from build123d import *

# Parameters (mm, degrees)
SKETCH_1_W          = 40
SKETCH_1_H          = 63
EXTRUDE_1_DEPTH     = 16
SKETCH_2_W          = 38
SKETCH_2_H          = 61
CUT_EXTRUDE_2_DEPTH = 15
FILLET_2_R          = 1
SKETCH_5_W          = 38
SKETCH_5_H          = 2
CUT_EXTRUDE_4_DEPTH = 0.5
SKETCH_6_W          = 61.5
SKETCH_6_H          = 2
CUT_EXTRUDE_5_DEPTH = 0.5
SKETCH_7_W          = 38.5
SKETCH_7_H          = 2
CUT_EXTRUDE_6_DEPTH = 0.5
SKETCH_8_W          = 62
SKETCH_8_H          = 2
CUT_EXTRUDE_7_DEPTH = 0.5


with BuildPart() as part:
    # Эскиз1 → Бобышка-Вытянуть1 (new body)
    with BuildSketch(Plane(origin=(0, 0, 0), x_dir=(1, 0, 0), z_dir=(0, 1, 0))):
        with Locations((18.915, -30.961)):
            Rectangle(SKETCH_1_W, SKETCH_1_H)
    extrude(amount=EXTRUDE_1_DEPTH)

    # Эскиз2 → Вырез-Вытянуть2 (cut)
    with BuildSketch(Plane(origin=(0, 16, 0), x_dir=(1, 0, 0), z_dir=(0, 1, 0))):
        with Locations((18.915, -30.961)):
            Rectangle(SKETCH_2_W, SKETCH_2_H)
    extrude(amount=-CUT_EXTRUDE_2_DEPTH, mode=Mode.SUBTRACT)

    # Скругление2
    fillet_2_edges = [part.edges().sort_by_distance(p)[0] for p in [
        (18.915, 0, -0.539),
        (38.915, 0, 30.961),
        (18.915, 0, 62.461),
        (-1.085, 0, 30.961),
    ]]
    fillet(fillet_2_edges, radius=FILLET_2_R)

    # Эскиз5 → Вырез-Вытянуть4 (cut)
    with BuildSketch(Plane(origin=(0, 0, 61.461), x_dir=(-1, 0, 0), z_dir=(0, 0, -1))):
        with Locations((-18.915, 15)):
            Rectangle(SKETCH_5_W, SKETCH_5_H)
    extrude(amount=-CUT_EXTRUDE_4_DEPTH, mode=Mode.SUBTRACT)

    # Эскиз6 → Вырез-Вытянуть5 (cut)
    with BuildSketch(Plane(origin=(-0.085, 0, 0), x_dir=(0, 0, -1), z_dir=(1, 0, 0))):
        with Locations((-31.211, 15)):
            Rectangle(SKETCH_6_W, SKETCH_6_H)
    extrude(amount=-CUT_EXTRUDE_5_DEPTH, mode=Mode.SUBTRACT)

    # Эскиз7 → Вырез-Вытянуть6 (cut)
    with BuildSketch(Plane.XY.offset(0.461)):
        with Locations((18.665, 15)):
            Rectangle(SKETCH_7_W, SKETCH_7_H)
    extrude(amount=-CUT_EXTRUDE_6_DEPTH, mode=Mode.SUBTRACT)

    # Эскиз8 → Вырез-Вытянуть7 (cut)
    with BuildSketch(Plane.ZY.offset(-37.915)):
        with Locations((30.961, 15)):
            Rectangle(SKETCH_8_W, SKETCH_8_H)
    extrude(amount=-CUT_EXTRUDE_7_DEPTH, mode=Mode.SUBTRACT)


solid = part.part
Geometry: final body of the model. Coordinates: model frame, mm. A direction names the side the tool comes from. Round coordinates to 2 decimals unless told otherwise and drop trailing zeros. Order: outer loops, then holes, each group sorted by start corner. A loop starts at its lowest first (then second) coordinate and runs counter-clockwise, first axis right, second up. Notation, with made-up numbers: (-33, 83.25) -> (21, 83.25) arc R20 cw to (21, 89.25) -> close; hole circle Ø8 at (-1, 2.5). An arc over 180 degrees is marked (long way). Put each result on its own line as item: value. Start each with the question number.
Q1. Line query: probe 1 along Z at (x, y) = (35, 2); probe 2 along X at (y, z) = (12.25, 28) (3 decimals); probe 3 along Y at (x, z) = (19, 55). Output: solid intervals per line, ascending.
Q2. Section B-B on z = 32.5. Return the cut outline in (x, y) (3 decimals).
Q3. Section A-A on y = 11.25. Return the cut outline in (x, z) (3 decimals).
Q4. First-contact query: pin 1 (5 mm diameter, centred on x = 24.5, z = 12.5, fed in from +Y). Flat tip, straight axial feed; report the tip coordinate or a pass-through.
Q5. Section C-C on x = 31.5. Return the cut outline in (y, z), and give its area (3 significant figures).
Q6. Reachability of faces 5 (the flat face through (38.915, 8, 31)), 6 (the flat face through (19, 15, 61.961)) from +Z, -Z, +X, -X, +Y, -Y: full face, straight path, thin tool, end or side. Return the list, or none.
Q7. Pull-direction query (Z, two-part tool) for faces 1 (the flat face through (19, 8, 0.461)), 2 (the flat face through (-1.085, 8, 31)), 3 (the flat face through (19, 8, 62.461)), 4 (the flat face through (19, 8, -0.539)); classes: +Z half, -Z half, draft (parallel to the pull), parting line (faces both ways), or undercut.
Ans:
1. probe 1: z = -0.54 to 0.46, 61.46 to 62.46
1. probe 2: x = -1.085 to -0.085, 37.915 to 38.915
1. probe 3: y = 0 to 1
2. outline: (-1.085, 1) arc R1 ccw to (-0.085, 0) -> (37.915, 0) arc R1 ccw to (38.915, 1) -> (38.915, 16) -> (38.415, 16) -> (38.415, 14) -> (37.915, 14) -> (37.915, 1) -> (-0.085, 1) -> (-0.085, 14) -> (-0.585, 14) -> (-0.585, 16) -> (-1.085, 16) -> close
3. outline: (-1.085, -0.539) -> (38.915, -0.539) -> (38.915, 62.461) -> (-1.085, 62.461) -> close; hole (-0.085, 0.461) -> (37.915, 0.461) -> (37.915, 61.461) -> (-0.085, 61.461) -> close
4. pin 1: stops at y = 1
5. outline: (0, 0.46) arc R1 ccw to (1, -0.54) -> (16, -0.54) -> (16, -0.04) -> (14, -0.04) -> (14, 0.46) -> (1, 0.46) -> (1, 61.46) -> (14, 61.46) -> (14, 61.96) -> (16, 61.96) -> (16, 62.46) -> (1, 62.46) arc R1 ccw to (0, 61.46) -> close
5. area: 90.6 mm2
6. face 5: +Z, -Z, +X, +Y, -Y
6. face 6: +Y
7. face 1: undercut
7. face 2: draft
7. face 3: +Z half
7. face 4: -Z half
